Autodesk Inventor part; units mm, degrees
ref_plane "YZ Plane" through (0, 0, 0) normal (1, 0, 0) x (0, 1, 0)
ref_plane "XZ Plane" through (0, 0, 0) normal (0, 1, 0) x (-1, 0, 0)
ref_plane "XY Plane" through (0, 0, 0) normal (0, 0, 1) x (1, 0, 0)
sketch "Sketch1" plane through (0, 0, 0) normal (0, 1, 0) x (-1, 0, 0)
  arc A0 (3.75, 6.4952) -> (3.75, -6.4952) centre (0, 0) ccw
  arc A1 (5.25, 9.0933) -> (5.25, -9.0933) centre (0, 0) ccw
  line L0 (-11.5, 15) -> (-24, 15)
  line L1 (-24, 15) -> (-24, -15)
  line L2 (-24, -15) -> (-11.5, -15)
  line L3 (-11.5, -15) -> (-11.5, 15)
  line L4 (-8.5, 18) -> (-27, 18)
  line L5 (-27, 18) -> (-27, -18)
  line L6 (-27, -18) -> (-8.5, -18)
  line L7 (-8.5, -18) -> (-8.5, 18)
  line L8 (0, 0) -> (5.25, 9.0933)
  line L9 (0, 0) -> (10.5, 0) construction
  line L10 (5.25, 9.0933) -> (0, 0)
  line L11 (0, 0) -> (5.25, -9.0933)
  line L12 (0, 0) -> (10.5, 0) construction
  dimension "d0" = 15
  dimension "d1" = 3
  dimension "d2" = 12.5
  dimension "d3" = 30
  dimension "d4" = 3
  dimension "d5" = 3
  dimension "d6" = 3
  dimension "d7" = 3
  dimension "d8" = 15
  dimension "d9" = 11.5
  dimension "d10" = 60
  dimension "d11" = 60
extrude "Extrusion1" add sketch "Sketch1" along normal blind 10 contours A0 L11 A1 L7 L8 | L7 A1 | A1 L7 L6 L5 L4
fillet "Fillet1" radius 2 4 edges at (-5.25, 5, 9.0933) (-3.75, 5, 6.4952) (-5.25, 5, -9.0933) (-3.75, 5, -6.4952)
fillet "Fillet2" radius 2 2 edges at (8.5, 5, 6.1644) (8.5, 5, -6.1644)
fillet "Fillet3" radius 1 4 edges at (8.5, 5, 18) (27, 5, 18) (8.5, 5, -18) (27, 5, -18)
sketch "Sketch2" plane through (0, 10, 0) normal (0, 1, 0) x (1, 0, 0)
  line L0 (11.5, -15) -> (11.5, 15)
  line L1 (11.5, 15) -> (24, 15)
  line L2 (24, 15) -> (24, -15)
  line L3 (24, -15) -> (11.5, -15)
  arc A0 (27, 17) -> (26, 18) centre (26, 17) ccw
  line L4 (26, 18) -> (9.5, 18)
  arc A1 (9.5, 18) -> (8.5, 17) centre (9.5, 17) ccw
  line L5 (8.5, 17) -> (8.5, 10.6771)
  arc A2 (5.46, 8.9687) -> (8.5, 10.6771) centre (6.5, 10.6771) ccw
  arc A3 (5.46, 8.9687) -> (-2.963, 10.0733) centre (0, 0) ccw
  arc A4 (-2.963, 10.0733) -> (-4.1307, 7.1545) centre (-2.3986, 8.1545) ccw
  arc A5 (-4.1307, 7.1545) -> (-2.5443, 7.0552) centre (-3.2228, 8.9366) ccw
  arc A6 (-2.5443, -7.0552) -> (-2.5443, 7.0552) centre (0, 0) ccw
  arc A7 (-2.5443, -7.0552) -> (-4.1307, -7.1545) centre (-3.2228, -8.9366) ccw
  arc A8 (-4.1307, -7.1545) -> (-2.963, -10.0733) centre (-2.3986, -8.1545) ccw
  arc A9 (-2.963, -10.0733) -> (5.46, -8.9687) centre (0, 0) ccw
  arc A10 (8.5, -10.6771) -> (5.46, -8.9687) centre (6.5, -10.6771) ccw
  line L6 (8.5, -10.6771) -> (8.5, -17)
  arc A11 (8.5, -17) -> (9.5, -18) centre (9.5, -17) ccw
  line L7 (9.5, -18) -> (26, -18)
  arc A12 (26, -18) -> (27, -17) centre (26, -17) ccw
  line L8 (27, -17) -> (27, 17)
  line L9 (11.5, 15) -> (24, 15)
  line L10 (24, 15) -> (24, 12)
  line L11 (24, 12) -> (11.5, 12)
  line L12 (11.5, 12) -> (11.5, 15)
  line L13 (11.5, -15) -> (24, -15)
  line L14 (24, -15) -> (24, -12)
  line L15 (24, -12) -> (11.5, -12)
  line L16 (11.5, -12) -> (11.5, -15)
  dimension "d17" = 3
  dimension "d18" = 3
extrude "Extrusion2" add sketch "Sketch2" against normal blind 1 contours L0 L15 L2 L3 | L0 L1 L2 L11
fillet "Fillet4" radius 2 4 edges at (11.5, 9.5, -12) (24, 9.5, -12) (11.5, 9.5, 12) (24, 9.5, 12)
equation "\"d5\" = d4"
equation "\"d6\" = d4"
equation "\"d7\" = d4"
properties part number "clip"
Source: CAD feature listing. Evaluate the final solid. Frame: model axes, mm. A direction names the side the tool comes from. Give positions to 0.01 mm unless a question says otherwise; leave off trailing zeros. Loops run counter-clockwise (first coordinate to the right, second up) from the corner with the lowest first, then second, coordinate; pieces in that order, holes last. Notation, with made-up numbers: (-1.75, 13.25) -> (16.25, 13.25) arc R13 cw to (16.25, 31.25) -> close; hole circle Ø6 at (-11.5, 65). An arc over 180 degrees is marked (long way). Use a Markdown table: item, result. Add a question column.
1) Line query: line 1 along Z through (x, y) = (0, 6.25); line 2 along X through (y, z) = (1.5, -9); line 3 along X through (y, z) = (7.5, 0). Output: solid intervals per line, ascending. Write a range as [from, to].
2) First-contact query: pin 1 (13.5 mm diameter, centred on x = 0, z = 0, fed in from +Y); pin 2 (3 mm diameter, centred on y = 5.5, z = -6, fed in from -X); pin 3 (5 mm diameter, centred on y = 2.5, z = -15.5, fed in from -X); pin 4 (5.5 mm diameter, centred on x = 20, z = 12, fed in from -Y). Flat tips, straight axial feed; report the tip coordinate or a pass-through.
3) Section query A-A, the plane z = 0. Return the cut outline in (x, y).
4) Section query C-C, the plane y = 4.25. Return the cut outline in (x, z).
5) Reachability of faces 5 (the face through (8.5, 5, 14)), 6 (the face through (7.454, 5.07, -8.919)), 7 (the face through (23.4, 9.49, -11.43)), 8 (the face through (18, 9, -14)) from +Z, -Z, +X, -X, +Y, -Y: full face, straight path, thin tool, end or side. Return the list, or none.
6) Pull-direction query (Z, two-part tool) for faces 1 (the face through (1.3, 4.93, -10.42)), 2 (the face through (18, 5, 18)), 3 (the face through (11.5, 5, 0)), 4 (the face through (11, 0, 1)); classes: +Z half, -Z half, draft (parallel to the pull), parting line (faces both ways), or undercut.
7) Section query D-D, the plane z = 13. Return the cut outline in (x, y).
8) Section query B-B, the plane x = 0. Return the cut outline in (y, z), then the cut area to 3 significant figures.
Numbers:
| question | item | result |
|---|---|---|
| 1 | line 1 | z = [-10.5, -7.5], [7.5, 10.5] |
| 1 | line 2 | x = [-4.21, 5.41], [7.59, 11.5], [24, 27] |
| 1 | line 3 | x = [7.5, 11.5], [24, 27] |
| 2 | pin 1 | passes through |
| 2 | pin 2 | stops at x = -4.29 |
| 2 | pin 3 | stops at x = 8.5 |
| 2 | pin 4 | stops at y = 9 |
| 3 | outline | (7.5, 0) -> (11.5, 0) -> (11.5, 10) -> (7.5, 10) -> close; (24, 0) -> (27, 0) -> (27, 10) -> (24, 10) -> close |
| 4 | outline | (-4.13, -7.15) arc R2 ccw to (-2.96, -10.07) arc R10.5 ccw to (5.46, -8.97) arc R2 cw to (8.5, -10.68) -> (8.5, -17) arc R1 ccw to (9.5, -18) -> (26, -18) arc R1 ccw to (27, -17) -> (27, 17) arc R1 ccw to (26, 18) -> (9.5, 18) arc R1 ccw to (8.5, 17) -> (8.5, 10.68) arc R2 cw to (5.46, 8.97) arc R10.5 ccw to (-2.96, 10.07) arc R2 ccw to (-4.13, 7.15) arc R2 ccw to (-2.54, 7.06) arc R7.5 cw (long way) to (-2.54, -7.06) arc R2 ccw to start; hole (11.5, -15) -> (24, -15) -> (24, 15) -> (11.5, 15) -> close |
| 5 | face 5 | +Z, -X, +Y, -Y |
| 5 | face 6 | -Z, +Y, -Y |
| 5 | face 7 | +Y, -Y |
| 5 | face 8 | -Y |
| 6 | face 1 | -Z half |
| 6 | face 2 | +Z half |
| 6 | face 3 | undercut |
| 6 | face 4 | draft |
| 7 | outline | (8.5, 0) -> (11.5, 0) -> (11.5, 9) -> (24, 9) -> (24, 0) -> (27, 0) -> (27, 10) -> (8.5, 10) -> close |
| 8 | outline | (0, -10.5) -> (10, -10.5) -> (10, -7.5) -> (0, -7.5) -> close; (0, 7.5) -> (10, 7.5) -> (10, 10.5) -> (0, 10.5) -> close |
| 8 | area | 60.0 mm2 |
